Read the model definition and answer for the solid it produces. Units are mm, in the model's axes. A direction names the side the tool comes from. Round coordinates to 2 decimals unless told otherwise and drop trailing zeros. Order: outer loops, then holes, each group sorted by start corner. A loop starts at its lowest first (then second) coordinate and runs counter-clockwise, first axis right, second up. Notation, with made-up numbers: (87.5, 37.25) - (146.5, 37.25) arc R28 cw to (146.5, 65.25) - close; hole circle Ø6 at (10.25, 89). An arc over 180 degrees is marked (long way). Answer as a JSON object with one key per item and string values. Group by question number.
Q1. A cutting plane is placed at A-A on z = 10.5. Determine the outline of the cut face in (x, y), and give its area (3 significant figures).
Q2. A cutting plane is placed at D-D on z = 2.75. Determine the outline of the cut face in (x, y), and give its area (3 significant figures).
Q3. A cutting plane is placed at B-B on y = -31. Determine the outline of the cut face in (x, z).
Q4. A cutting plane is placed at C-C on x = 37. Determine the outline of the cut face in (y, z).
Q5. Consider line 1 (X direction, y = 49, z = 11.25); line 2 (Y direction, x = 22, z = 9.75); line 3 (Z direction, x = 12, y = 45). Determine where each line is inside the solid, lowest interval first.
Q6. Given pin 1 Ø1 at (x, y) = (35, 47) entering from +Z; pin 2 Ø1.5 at (x, z) = (2, 1.5) entering from +Y, each flat-ended and moving along its own axis, determine where each tip first touches the part or whether it passes through.
Q7. A tool of negligible diameter and unlimited length cuts with its end or side. For faces 5 (the flat face through (41.319, -1, 8)), 6 (the flat face through (-43.859, -1, 9)), from which of +Z, -Z, +X, -X, +Y, -Y can it reach the whole face along a straight path? Write none if from no direction.
Q8. The mould has two halves that part along Y. Classify faces 1 (the flat face through (-1, -76.713, 9)), 2 (the flat face through (-1, -74.173, 8)), 3 (the flat face through (-1, 76.713, 9)), 4 (the cylindrical face through (-42.41, 1.07, 1.53)): pulls with the +Y half, pulls with the -Y half, needs draft (parallel to the pull), parting line crosses it, or undercut.
```python
from build123d import *

# Parameters (mm, degrees)
F0_W     = 87.7170339227
F0_H     = 153.4254997969
F1_DEPTH = 1.7726365477
F2_W     = 87.7170339227
F2_H     = 153.4254997969
F3_DEPTH = 5.9710852802
F4_T     = -2.54
F5_DEPTH = 4.318
F6_R     = 5.08


with BuildPart() as f1:
    # F0 (on Top) → F1 (new body)
    with BuildSketch(Plane.XY):
        Rectangle(F0_W, F0_H)
    extrude(amount=F1_DEPTH)

    # F2 (on face) → F3 (join)
    with BuildSketch(Plane.XY.offset(1.7726365477)):
        Rectangle(F2_W, F2_H)
    extrude(amount=F3_DEPTH)

    # F4
    f4_openings = [f1.faces().sort_by_distance(p)[0] for p in [
        (0, 0, 7.743722),
    ]]
    offset(amount=F4_T, openings=f4_openings)

    # F5 (add): faces of the model
    f5_faces = [f1.faces().sort_by_distance(p)[0] for p in [
        (-42.0912121764, 0, 7.7437218279),
        (0, 0, 0),
    ]]
    extrude(f5_faces, amount=F5_DEPTH, dir=(0, 0, 1))

    # F6
    f6_edges = [f1.edges().sort_by_distance(p)[0] for p in [
        (0, -76.71275, 0),
        (43.858517, 0, 0),
        (0, 76.71275, 0),
        (-43.858517, 0, 0),
    ]]
    fillet(f6_edges, radius=F6_R)


solid = f1.part
```
Result set:
{
 "1": {"outline": "(-43.86, -76.71) - (43.86, -76.71) - (43.86, 76.71) - (-43.86, 76.71) - close; hole (-41.32, -74.17) - (41.32, -74.17) - (41.32, 74.17) - (-41.32, 74.17) - close", "area": "1,200 mm²"},
 "2": {"outline": "(-43.29, -76.15) - (43.29, -76.15) - (43.29, 76.15) - (-43.29, 76.15) - close", "area": "13,200 mm²"},
 "3": {"outline": "(-43.86, 5.08) arc R5.08 ccw to (-38.78, 0) - (38.78, 0) arc R5.08 ccw to (43.86, 5.08) - (43.86, 12.06) - (41.32, 12.06) - (41.32, 4.32) - (-41.32, 4.32) - (-41.32, 12.06) - (-43.86, 12.06) - close"},
 "4": {"outline": "(-76.71, 5.08) arc R5.08 ccw to (-71.63, 0) - (71.63, 0) arc R5.08 ccw to (76.71, 5.08) - (76.71, 12.06) - (74.17, 12.06) - (74.17, 4.32) - (-74.17, 4.32) - (-74.17, 12.06) - (-76.71, 12.06) - close"},
 "5": {"line 1": "x = -43.86 to -41.32, 41.32 to 43.86", "line 2": "y = -76.71 to -74.17, 74.17 to 76.71", "line 3": "z = 0 to 4.32"},
 "6": {"pin 1": "stops at z = 4.32", "pin 2": "stops at y = 75.85"},
 "7": {"face 5": "+Z", "face 6": "+Z, -Z, -X, +Y, -Y"},
 "8": {"face 1": "pulls with the -Y half", "face 2": "undercut", "face 3": "pulls with the +Y half", "face 4": "needs draft"}
}
